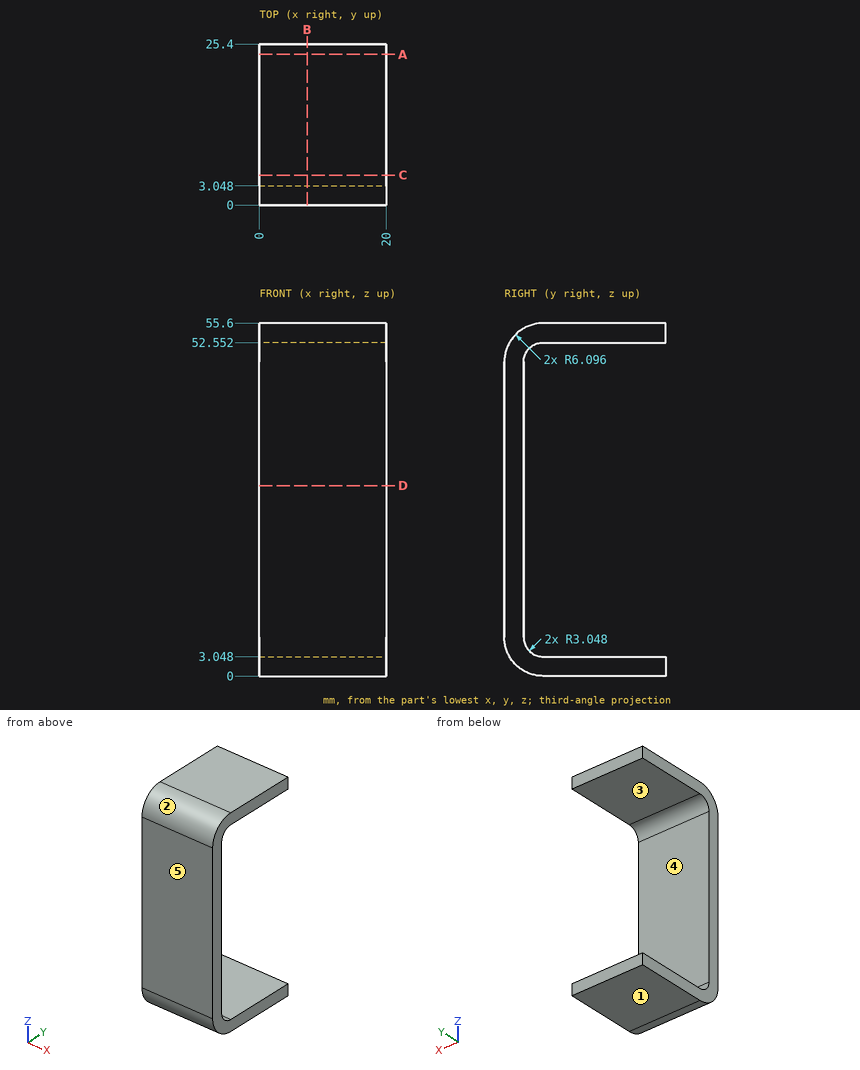
Could you check a few things on this drawing? It's one solid part, dimensions in mm from its lowest x, y, z. A direction names the side the tool comes from. Give positions to 0.01 mm unless a question says otherwise; leave off trailing zeros. Write each loop counter-clockwise with the first axis right and the second up, starting at its lowest first coordinate (ties: lowest second). Pieces come first, ordered by that corner, then holes.
(1) If I drill on L1, parallel to Z at x = 9, y = 19.75; L2, parallel to Y at x = 12, z = 21.5; L3, parallel to Y at x = 2.75, z = 3, over which ranges is the centre line in solid material (lowest first)?
Output values:
L1: z = 0 to 3.05, 52.55 to 55.6
L2: y = 0 to 3.05
L3: y = 0.84 to 25.4
(2) Will this pin go through, and if not, where does the flat tip stop? pin 1 (3 mm diameter, centred on x = 8, z = 42, fed in from +Y).
Output values:
pin 1: stops at y = 3.05
(3) Imagine slicing it at A-A, the plane y = 23.75. Write out the boundary of the cut face in (x, z), and give its area (3 significant figures).
Output values:
outline: (0, 0) - (20, 0) - (20, 3.05) - (0, 3.05) - close; (0, 52.55) - (20, 52.55) - (20, 55.6) - (0, 55.6) - close
area: 122 mm2
(4) Imagine slicing it at C-C, the plane y = 4.75. Write out the boundary of the cut face in (x, z).
Output values:
outline: (0, 0.15) - (20, 0.15) - (20, 3.36) - (0, 3.36) - close; (0, 52.24) - (20, 52.24) - (20, 55.45) - (0, 55.45) - close
(5) On a 3-axis mill with a long thin cutter (end or side, diameter ignored), from which of +Z, -Z, +X, -X, +Y, -Y can I reach the whole of each face in a straight line? I mean the marked faces 4 and 5. Say none if no direction works.
Output values:
face 4: +X, -X, +Y
face 5: +Z, -Z, +X, -X, -Y
(6) Imagine slicing it at B-B, the plane x = 7.5. Write out the boundary of the cut face in (y, z).
Output values:
outline: (0, 6.1) arc R6.1 ccw to (6.1, 0) - (25.4, 0) - (25.4, 3.05) - (6.1, 3.05) arc R3.05 cw to (3.05, 6.1) - (3.05, 49.5) arc R3.05 cw to (6.1, 52.55) - (25.4, 52.55) - (25.4, 55.6) - (6.1, 55.6) arc R6.1 ccw to (0, 49.5) - close
(7) Imagine slicing it at D-D, the plane z = 30. Write out the boundary of the cut face in (x, y).
Output values:
outline: (0, 0) - (20, 0) - (20, 3.05) - (0, 3.05) - close
(8) Thinking about a two-plate mould opening in Z: for the marked faces 1, 2 and 3, which applies, pulls with the +Z half, pulls with the -Z half, needs draft (parallel to the pull), parting line crosses it, or undercut?
Output values:
face 1: pulls with the -Z half
face 2: pulls with the +Z half
face 3: undercut
